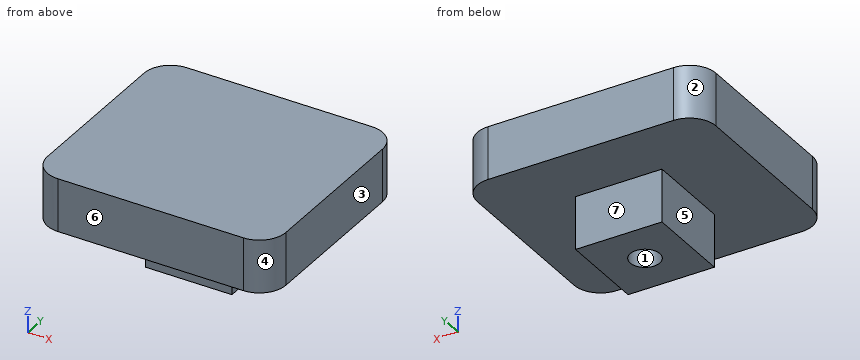
from build123d import *

# Parameters (mm, degrees)
EXTRUDE_1_DEPTH     = 25.4
SKETCH_2_W          = 41.402
SKETCH_2_H          = 41.402
EXTRUDE_2_DEPTH     = 25.4
SKETCH_3_R          = 7.112
CUT_EXTRUDE_1_DEPTH = 25.4


with BuildPart() as part:
    # 草图1 → 凸台-拉伸1 (new body)
    with BuildSketch(Plane.XY):
        with BuildLine():
            Line((12.7, 0), (101.6, 0))
            ThreePointArc((101.6, 0), (110.580256121, 3.719743879), (114.3, 12.7))
            Line((114.3, 12.7), (114.3, 88.9))
            ThreePointArc((114.3, 88.9), (110.580256121, 97.880256121), (101.6, 101.6))
            Line((101.6, 101.6), (12.7, 101.6))
            ThreePointArc((12.7, 101.6), (3.719743879, 97.880256121), (0, 88.9))
            Line((0, 88.9), (0, 12.7))
            ThreePointArc((0, 12.7), (3.719743879, 3.719743879), (12.7, 0))
        make_face()
    extrude(amount=EXTRUDE_1_DEPTH)

    # 草图2 → 凸台-拉伸2 (add)
    with BuildSketch(Plane(origin=(0, 0, 0), x_dir=(-1, 0, 0), z_dir=(0, 0, -1))):
        with Locations((-57.15, 50.8)):
            Rectangle(SKETCH_2_W, SKETCH_2_H)
    extrude(amount=EXTRUDE_2_DEPTH)

    # 草图3 → 切除-拉伸1 (cut)
    with BuildSketch(Plane(origin=(0, 0, -25.4), x_dir=(-1, 0, 0), z_dir=(0, 0, -1))):
        with Locations((-57.15, 50.8)):
            Circle(SKETCH_3_R)
    extrude(amount=-CUT_EXTRUDE_1_DEPTH, mode=Mode.SUBTRACT)


solid = part.part
Read the model definition and answer for the solid it produces. Units are mm, in the model's axes. Face numbers are marked on the shaded views. A direction names the side the tool comes from. Coordinates: 2 decimals unless noted, no trailing zeros. Loops run counter-clockwise (first coordinate to the right, second up) from the corner with the lowest first, then second, coordinate; pieces in that order, holes last. Notation, with made-up numbers: (7, -23) - (58, -23) arc R14 ccw to (58, -8) - close; hole circle Ø6 at (18, 14.5). An arc over 180 degrees is marked (long way). Answer in a Markdown table with one row per item.
Q1. Find section A-A on x = 57.15. Write down the section's boundary in (y, z), plus the area to 3 significant figures.
Here are the results:
| item | result |
|---|---|
| outline | (0, 0) - (30.1, 0) - (30.1, -25.4) - (43.69, -25.4) - (43.69, 0) - (57.91, 0) - (57.91, -25.4) - (71.5, -25.4) - (71.5, 0) - (101.6, 0) - (101.6, 25.4) - (0, 25.4) - close |
| area | 3,270 mm^2 |
Q2. Given P1, Ø20.5, axis at x = 51, z = -18.5, coming from the -Y side; P2, Ø1, axis at x = 57, z = -12.5, coming from the +Y side; P3, Ø2, axis at y = 59, z = -8, coming from the +X side, each flat-ended and moving along its own axis, determine where each tip first touches the part or whether it passes through.
Here are the results:
| item | result |
|---|---|
| P1 | stops at y = 30.1 |
| P2 | stops at y = 71.5 |
| P3 | stops at x = 77.85 |
Q3. The mould has two halves that part along Y. Classify the marked faces 1, 2, 3 and 4: pulls with the +Y half, pulls with the -Y half, needs draft (parallel to the pull), parting line crosses it, or undercut.
Here are the results:
| item | result |
|---|---|
| face 1 | undercut |
| face 2 | pulls with the +Y half |
| face 3 | needs draft |
| face 4 | pulls with the -Y half |
Q4. Find section B-B on z = -6. Write down the section's boundary in (x, y), plus the area to 3 significant figures.
Here are the results:
| item | result |
|---|---|
| outline | (36.45, 30.1) - (77.85, 30.1) - (77.85, 71.5) - (36.45, 71.5) - close; hole circle Ø14.22 at (57.15, 50.8) |
| area | 1,560 mm^2 |
Q5. For the marked faces 5, 6 and 7, determine the directions among +Z, -Z, +X, -X, +Y, -Y from which every point of the face is accessible in a straight line to the end or side of a thin tool.
Here are the results:
| item | result |
|---|---|
| face 5 | -Z, -X, +Y, -Y |
| face 6 | +Z, -Z, +X, -X, -Y |
| face 7 | -Z, +X, -X, +Y |
Q6. Find section C-C on y = 50.8. Write down the section's boundary in (x, z).
Here are the results:
| item | result |
|---|---|
| outline | (0, 0) - (36.45, 0) - (36.45, -25.4) - (50.04, -25.4) - (50.04, 0) - (64.26, 0) - (64.26, -25.4) - (77.85, -25.4) - (77.85, 0) - (114.3, 0) - (114.3, 25.4) - (0, 25.4) - close |
Q7. Straight lines are drawn through the part: line 1 along Y through (x, z) = (57.15, -16.75); line 2 along Z through (x, y) = (7, 7); line 3 along X through (y, z) = (57, -12.5). For each, find the intervals that lie inside material, in ascending order. Write a range as [from, to].
Here are the results:
| item | result |
|---|---|
| line 1 | y = [30.1, 43.69], [57.91, 71.5] |
| line 2 | z = [0, 25.4] |
| line 3 | x = [36.45, 53.67], [60.63, 77.85] |
Q8. Find section D-D on y = 16. Write down the section's boundary in (x, z), plus the area to 3 significant figures.
Here are the results:
| item | result |
|---|---|
| outline | (0, 0) - (114.3, 0) - (114.3, 25.4) - (0, 25.4) - close |
| area | 2,900 mm^2 |
